```python
from build123d import *
from build123d.topology import SkipClean

# Parameters (mm, degrees)
CROQUIS1_R                      = 1.5
CROQUIS1_R_2                    = 1.625
SALIENTE_EXTRUIR1_DEPTH         = 2.5
SALIENTE_EXTRUIR2_START         = 1.58
CROQUIS2_R                      = 1.625
SALIENTE_EXTRUIR2_DEPTH         = 1.58
CROQUIS3_R                      = 3.35997123
CORTAR_EXTRUIR1_DEPTH           = 1.8
CORTAR_EXTRUIR1_DRAFT           = -46
CORTAR_EXTRUIR1_PROFILE_2_DEPTH = 1.8
CORTAR_EXTRUIR1_PROFILE_2_DRAFT = -46


with BuildPart() as part:
    # Croquis1 → Saliente-Extruir1 (new body)
    with BuildSketch(Plane.XY):
        Polygon((-90.077371, -80.148646), (-88.732371, -81.493646), (-75.732371, -81.493646), (-75.732371, -74.071146), (-83.98707047, -66.648646), (-88.732371, -66.648646), (-96.232371, -66.648646), (-96.232371, -80.148646), align=None)
        with Locations((-92.232371, -75.223646)):
            Circle(CROQUIS1_R, mode=Mode.SUBTRACT)
        with Locations((-79.72767153, -75.223646)):
            Circle(CROQUIS1_R_2, mode=Mode.SUBTRACT)
    extrude(amount=SALIENTE_EXTRUIR1_DEPTH)

    # Croquis2 → Saliente-Extruir2 (add)
    with SkipClean():  # the faces are left unmerged after this step: merging them gives an invalid solid
        with BuildSketch(Plane(origin=(0, 0, 0), x_dir=(-1, 0, 0), z_dir=(0, 0, -1)).offset(SALIENTE_EXTRUIR2_START)):
            Polygon((75.732371, -74.071146), (75.732371, -80.148646), (88.732371, -80.148646), (88.732371, -66.648646), (83.98707047, -66.648646), align=None)
            with Locations((79.72767153, -75.223646)):
                Circle(CROQUIS2_R, mode=Mode.SUBTRACT)
        extrude(amount=-SALIENTE_EXTRUIR2_DEPTH)


with BuildPart() as cortar_extruir1_tool:
    # Croquis3 → Cortar-Extruir1 (with draft: the straight prism first)
    with BuildSketch(Plane.XY.offset(2.5)):
        with Locations((-92.232371, -75.223646)):
            Circle(CROQUIS3_R)
    extrude(amount=-CORTAR_EXTRUIR1_DEPTH)
    # Cortar-Extruir1: the draft: its side faces are tilted about the plane it starts from
    cortar_extruir1_sides = [cortar_extruir1_tool.faces().sort_by_distance(p)[0] for p in [
        (-95.59234223, -75.223646, 1.6),
    ]]
    draft(cortar_extruir1_sides, Plane.XY.offset(2.5), CORTAR_EXTRUIR1_DRAFT)


with BuildPart() as part_1:
    add(part.part)

    # Cortar-Extruir1: cut by cortar_extruir1_tool
    add(cortar_extruir1_tool.part, mode=Mode.SUBTRACT)


with BuildPart() as cortar_extruir1_profile_2_tool:
    # Croquis3 → Cortar-Extruir1 profile 2 (with draft: the straight prism first)
    with BuildSketch(Plane.XY.offset(2.5)):
        with Locations((-79.72767153, -75.223646)):
            Circle(CROQUIS3_R)
    extrude(amount=-CORTAR_EXTRUIR1_PROFILE_2_DEPTH)
    # Cortar-Extruir1 profile 2: the draft: its side faces are tilted about the plane it starts from
    cortar_extruir1_profile_2_sides = [cortar_extruir1_profile_2_tool.faces().sort_by_distance(p)[0] for p in [
        (-83.08764276, -75.223646, 1.6),
    ]]
    draft(cortar_extruir1_profile_2_sides, Plane.XY.offset(2.5), CORTAR_EXTRUIR1_PROFILE_2_DRAFT)


with BuildPart() as part_2:
    add(part_1.part)

    # Cortar-Extruir1 profile 2: cut by cortar_extruir1_profile_2_tool
    add(cortar_extruir1_profile_2_tool.part, mode=Mode.SUBTRACT)


solid = part_2.part
```
Work out the finished part from the listing and answer in its coordinate system (mm). A direction names the side the tool comes from. Give positions to 0.01 mm unless a question says otherwise; leave off trailing zeros. Loops run counter-clockwise (first coordinate to the right, second up) from the corner with the lowest first, then second, coordinate; pieces in that order, holes last. Notation, with made-up numbers: (54.5, 84.25) -> (90.5, 84.25) arc R29 cw to (90.5, 113.25) -> close; hole circle Ø5 at (35, 19). An arc over 180 degrees is marked (long way). Write item = value, one per line. Start each with the question number.
(1) Find section D-D on z = -1.3. Give the vertices of the cut face in (x, y) (3 decimals).
(2) Which of the six approach directions +Z, -Z, +X, -X, +Y, -Y give full straight-line access (tool end or side, diameter ignored) to faces 1 (the flat face through (-82, -80.149, -1)), 2 (the flat face through (-93, -80.149, 1)), 3 (the flat face through (-88.732, -73, -1)), 4 (the cylindrical face through (-91.426, -73.959, 0.347)), 5 (the flat face through (-82, -81.494, 1))?
(3) Find section B-B on z = 1.85. Give the vertices of the cut face in (x, y).
(4) Find the intervals of material crossed by probe 1 along X at (y, z) = (-73, 1.75); probe 2 along X at (y, z) = (-74.75, 0.1); probe 3 along X at (y, z) = (-73.5, -0.3), in increasing order. Write a range as from..to.
(5) Find section C-C on y = -70. Give the vertices of the cut face in (x, z).
(6) The mould has two halves that part along X. Classify faces 6 (the flat face through (-90.6, -74.6, 0)), 7 (the flat face through (-96.232, -73, 1)), 8 (the flat face through (-79.918, -70.308, 0.431)), 9 (the conical face through (-93.424, -74.131, 0.816)): +X half, -X half, draft (parallel to the pull), parting line (faces both ways), or undercut.
(7) Find section A-A on x = -85. Give the vertices of the cut face in (y, z), and give its area (3 significant figures).
(8) Given pin 1 Ø3.5 at (x, y) = (-79.73, -75.22) entering from +Z; pin 2 Ø1.3 at (x, z) = (-80, -0.5) entering from -Y; pin 3 Ø1.7 at (y, z) = (-74, -1) entering from -X; pin 4 Ø6 at (x, y) = (-94, -72) entering from -Z, each flat-ended and moving along its own axis, determine where each tip first touches the part or whether it passes through.
From the geometry:
q1.outline = (-88.732, -80.149) -> (-75.732, -80.149) -> (-75.732, -74.071) -> (-83.987, -66.649) -> (-88.732, -66.649) -> close; hole circle Ø3.25 at (-79.728, -75.224)
q2.face_1 = -Z, +X, -X, -Y
q2.face_2 = +Z, -Z, -X, -Y
q2.face_3 = -Z, -X, +Y, -Y
q2.face_4 = +Z, -Z
q2.face_5 = +Z, -Z, +X, -X, -Y
q3.outline = (-96.23, -80.15) -> (-90.08, -80.15) -> (-88.73, -81.49) -> (-75.73, -81.49) -> (-75.73, -74.07) -> (-83.99, -66.65) -> (-96.23, -66.65) -> close; hole circle Ø5.37 at (-92.23, -75.22); hole circle Ø5.37 at (-79.73, -75.22)
q4.probe_1 = -96.23..-93.55, -90.92..-81.04, -78.41..-76.92
q4.probe_2 = -96.23..-93.66, -90.81..-81.28, -78.17..-75.73
q4.probe_3 = -88.73..-76.37
q5.outline = (-96.23, 0) -> (-88.73, 0) -> (-88.73, -1.58) -> (-80.26, -1.58) -> (-80.26, 2.5) -> (-96.23, 2.5) -> close
q6.face_6 = draft
q6.face_7 = -X half
q6.face_8 = +X half
q6.face_9 = undercut
q7.outline = (-81.49, 0) -> (-80.15, 0) -> (-80.15, -1.58) -> (-66.65, -1.58) -> (-66.65, 2.5) -> (-81.49, 2.5) -> close
q7.area = 58.4 mm^2
q8.pin_1 = 0.95
q8.pin_2 = -81.49
q8.pin_3 = -88.73
q8.pin_4 = 0
